```python
from build123d import *

# Parameters (mm, degrees)
ESTRUSIONE_ESTRUSIONE1_DEPTH = 39
FORO_PER_VITE_M8_1_D         = 9
FORO_PER_VITE_M8_1_DEPTH     = 30
FORO_PER_VITE_M8_1_TIP       = 2.703872786
RACCORDO1_R                  = 1.5


with BuildPart() as part:
    # Schizzo1 → Estrusione-Estrusione1 (new body)
    with BuildSketch(Plane.XY):
        with BuildLine():
            Line((-21.5, 15), (-22.5, 0))
            Line((-22.5, 0), (22.5, 0))
            Line((22.5, 0), (21.5, 15))
            Line((21.5, 15), (8.5, 15))
            ThreePointArc((8.5, 15), (7.984359711, 12.084524053), (6.5, 9.522774425))
            Line((6.5, 9.522774425), (-6.5, 9.522774425))
            ThreePointArc((-6.5, 9.522774425), (-7.984359711, 12.084524053), (-8.5, 15))
            Line((-8.5, 15), (-21.5, 15))
        make_face()
    extrude(amount=ESTRUSIONE_ESTRUSIONE1_DEPTH)

    # Foro per Vite M8-1
    with Locations(Plane(origin=(0, 0, 0), x_dir=(-1, 0, 0), z_dir=(0, -1, 0))):
        with Locations((-15.5, -31.5), (15.5, -31.5), (15.5, -7.5), (-15.5, -7.5)):
            Hole(FORO_PER_VITE_M8_1_D / 2, depth=FORO_PER_VITE_M8_1_DEPTH)
            with Locations((0, 0, -(FORO_PER_VITE_M8_1_DEPTH + FORO_PER_VITE_M8_1_TIP / 2))):  # 118° drill point
                Cone(0, FORO_PER_VITE_M8_1_D / 2, FORO_PER_VITE_M8_1_TIP, mode=Mode.SUBTRACT)

    # Raccordo1
    raccordo1_edges = [part.edges().sort_by_distance(p)[0] for p in [
        (22, 7.5, 0),
        (-22, 7.5, 0),
        (22, 7.5, 39),
        (-22, 7.5, 39),
    ]]
    fillet(raccordo1_edges, radius=RACCORDO1_R)


solid = part.part
```
Check sheet for the modelled part. Datum: model origin and axes. Units: mm. A direction names the side the tool comes from. Coordinates: 2 decimals unless noted, no trailing zeros. Order: outer loops, then holes, each group sorted by start corner. A loop starts at its lowest first (then second) coordinate and runs counter-clockwise, first axis right, second up. Notation, with made-up numbers: (67, 39) -> (91, 39) arc R10 cw to (91, 56) -> close; hole circle Ø6 at (-10.75, -8). An arc over 180 degrees is marked (long way). Write each question's results on one line, items separated by ' | '. Start each with the question number.
1) Section check B-B (z = 31.5). Enter the section's corners in (x, y), and give its area (3 significant figures).
2) Section check C-C (z = 26.5). Enter the section's corners in (x, y), and give its area (3 significant figures).
3) Section check D-D (y = 13). Count the separate pieces of the cut face and the enclosed holes in it, and give its area (3 significant figures).
4) Section check A-A (x = -15.5). Enter the section's corners in (y, z).
5) Draft check along Z on faces 1 (the face through (0, 9.523, 19)), 2 (the face through (-21.577, 7.416, 0.451)), 3 (the face through (-16.48, 7.61, 35.89)). Enter one of: pulls with the +Z half, pulls with the -Z half, needs draft (parallel to the pull), parting line crosses it, or undercut.
6) Set-up check for faces 4 (the face through (-15, 15, 19)), 5 (the face through (-7.97, 12.05, 19.23)): record each of +Z, -Z, +X, -X, +Y, -Y from which the full face is reachable in a straight line by a thin tool's end or side.
7) Material ranges on line 1 along Z through (x, y) = (15.5, 7.5); line 2 along Z through (x, y) = (-13, 14); line 3 along X through (y, z) = (6.75, 10), recorded low to high.
8) Depth check by flat-ended pin: pin 1 (1.5 mm diameter, centred on x = 1, z = 18, fed in from +Y); pin 2 (7 mm diameter, centred on x = -15.5, z = 31.5, fed in from -Y); pin 3 (2 mm diameter, centred on y = 6, z = 24, fed in from -X). Enter the tip coordinate at first touch or a pass-through.
Checked values:
1) outline: (-22.5, 0) -> (-20, 0) -> (-20, 15) -> (-21.5, 15) -> close; (-11, 0) -> (11, 0) -> (11, 15) -> (8.5, 15) arc R8.5 cw to (6.5, 9.52) -> (-6.5, 9.52) arc R8.5 cw to (-8.5, 15) -> (-11, 15) -> close; (20, 0) -> (22.5, 0) -> (21.5, 15) -> (20, 15) -> close | area: 304 mm²
2) outline: (-22.5, 0) -> (22.5, 0) -> (21.5, 15) -> (8.5, 15) arc R8.5 cw to (6.5, 9.52) -> (-6.5, 9.52) arc R8.5 cw to (-8.5, 15) -> (-21.5, 15) -> close | area: 574 mm²
3) separate pieces: 2 | enclosed holes: 4 | area: 787 mm²
4) outline: (0, 0) -> (15, 0) -> (15, 3) -> (0, 3) -> close; (0, 12) -> (15, 12) -> (15, 27) -> (0, 27) -> close; (0, 36) -> (15, 36) -> (15, 39) -> (0, 39) -> close
5) face 1: needs draft | face 2: pulls with the -Z half | face 3: undercut
6) face 4: +Z, -Z, +X, -X, +Y | face 5: +Z, -Z, +Y
7) line 1: 0 to 3, 12 to 27, 36 to 39 | line 2: 0 to 3.76, 11.24 to 27.76, 35.24 to 39 | line 3: -22.05 to -19.24, -11.76 to 11.76, 19.24 to 22.05
8) pin 1: y = 9.52 | pin 2: through | pin 3: x = -22.17
